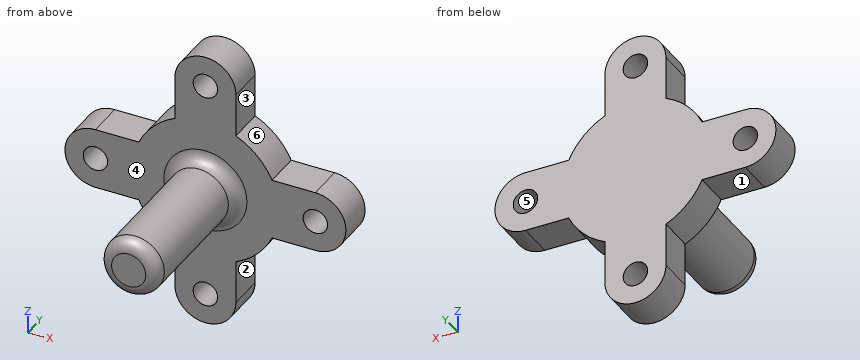
```python
from build123d import *

# Parameters (mm, degrees)
SKETCH1_R           = 5
BOSS_EXTRUDE1_DEPTH = 7.5
SKETCH2_R           = 12
BOSS_EXTRUDE2_DEPTH = 60
FILLET1_R           = 5
SCALE1_SCALE        = 0.6


with BuildPart() as part:
    # Sketch1 → Boss-Extrude1 (new body, symmetric)
    with BuildSketch(Plane(origin=(0, 0, 0), x_dir=(1, 0, 0), z_dir=(0, 1, 0))):
        with BuildLine():
            Line((12.5, 45.011324124), (12.5, 27.271780287))
            ThreePointArc((12.5, 27.271780287), (21.213203436, 21.213203436), (27.271780287, 12.5))
            Line((27.271780287, 12.5), (45, 12.5))
            ThreePointArc((45, 12.5), (57.511322842, 0.00566206), (45.011324124, -12.5))
            Line((45.011324124, -12.5), (27.271780287, -12.5))
            ThreePointArc((27.271780287, -12.5), (21.213203436, -21.213203436), (12.5, -27.271780287))
            Line((12.5, -27.271780287), (12.5, -45))
            ThreePointArc((12.5, -45), (0.00566206, -57.511322842), (-12.5, -45.011324124))
            Line((-12.5, -45.011324124), (-12.5, -27.271780287))
            ThreePointArc((-12.5, -27.271780287), (-21.213203436, -21.213203436), (-27.271780287, -12.5))
            Line((-27.271780287, -12.5), (-45, -12.5))
            ThreePointArc((-45, -12.5), (-57.511322842, -0.00566206), (-45.011324124, 12.5))
            Line((-45.011324124, 12.5), (-27.271780287, 12.5))
            ThreePointArc((-27.271780287, 12.5), (-21.213203436, 21.213203436), (-12.5, 27.271780287))
            Line((-12.5, 27.271780287), (-12.5, 45))
            ThreePointArc((-12.5, 45), (-0.00566206, 57.511322842), (12.5, 45.011324124))
        make_face()
        with Locations((0, 45.011324124)):
            Circle(SKETCH1_R, mode=Mode.SUBTRACT)
        with Locations((45.011324124, 0)):
            Circle(SKETCH1_R, mode=Mode.SUBTRACT)
        with Locations((0, -45.011324124)):
            Circle(SKETCH1_R, mode=Mode.SUBTRACT)
        with Locations((-45.011324124, 0)):
            Circle(SKETCH1_R, mode=Mode.SUBTRACT)
    extrude(amount=BOSS_EXTRUDE1_DEPTH, both=True)

    # Sketch2 → Boss-Extrude2 (add)
    with BuildSketch(Plane.XZ.offset(7.5)):
        Circle(SKETCH2_R)
    extrude(amount=BOSS_EXTRUDE2_DEPTH)

    # Fillet1
    fillet1_edges = [part.edges().sort_by_distance(p)[0] for p in [
        (-12, -7.5, 0),
        (-12, -67.5, 0),
    ]]
    fillet(fillet1_edges, radius=FILLET1_R)


with BuildPart() as part_1:
    # Scale1: scaled about (0, -9.636129327, 0)
    add(part.part.scale(SCALE1_SCALE).moved(Location((0, -3.854451731, 0))))


solid = part_1.part
```
Check sheet for the modelled part. Datum: model origin and axes. Units: mm. Face numbers are marked on the shaded views. A direction names the side the tool comes from. Round coordinates to 2 decimals unless told otherwise and drop trailing zeros. Loops run counter-clockwise (first coordinate to the right, second up) from the corner with the lowest first, then second, coordinate; pieces in that order, holes last. Notation, with made-up numbers: M 36,19.25 L 40,19.25 A20 cw 40,49.25 Z; hole C -2.5,79.25 d11. An arc over 180 degrees is marked long. Answer as a JSON object with one key per item and string values.
1. Section check B-B (z = -25.5). Record the boundary of the cut face in (x, y).
Reply:
{"outline": "M -7.5,-8.35 L -2.59,-8.35 L -2.59,0.65 L -7.5,0.65 Z; M 2.59,-8.35 L 7.5,-8.35 L 7.5,0.65 L 2.59,0.65 Z"}
2. Scan lines: line 1 (Z direction, x = 0, y = -4.75); line 2 (X direction, y = -1, z = 2). Record each from-to range of solid material in increasing order.
Reply:
{"line 1": "z = -34.51 to -30.01, -24.01 to 24.01, 30.01 to 34.51", "line 2": "x = -34.24 to -29.24, -24.77 to 24.77, 29.24 to 34.24"}
3. Access from +Z, -Z, +X, -X, +Y, -Y to the whole of each face (thin tool, end or side, straight path). Record for the marked faces 1, 2 and 3.
Reply:
{"face 1": "-Z, -X, +Y, -Y", "face 2": "-Z, +X, +Y, -Y", "face 3": "+Z, +X, +Y, -Y"}
4. Section check D-D (y = -15). Record the boundary of the cut face in (x, z).
Reply:
{"outline": "C 0,0 d14.4"}
5. Mould release check, pull along X, two halves, no side actions. Record for the marked faces 4, 5 and 6: pulls with the +X half, pulls with the -X half, needs draft (parallel to the pull), parting line crosses it, or undercut.
Reply:
{"face 4": "needs draft", "face 5": "undercut", "face 6": "pulls with the +X half"}
6. Section check A-A (x = 0). Record the boundary of the cut face in (y, z).
Reply:
{"outline": "M -44.35,-4.2 A3 ccw -41.35,-7.2 L -11.35,-7.2 A3 cw -8.35,-10.2 L -8.35,-24.01 L 0.65,-24.01 L 0.65,24.01 L -8.35,24.01 L -8.35,10.2 A3 cw -11.35,7.2 L -41.35,7.2 A3 ccw -44.35,4.2 Z; M -8.35,-34.51 L 0.65,-34.51 L 0.65,-30.01 L -8.35,-30.01 Z; M -8.35,30.01 L 0.65,30.01 L 0.65,34.51 L -8.35,34.51 Z"}
7. Section check C-C (z = 0). Record the boundary of the cut face in (x, y), plus the area to 3 significant figures.
Reply:
{"outline": "M -34.51,-8.35 L -30.01,-8.35 L -30.01,0.65 L -34.51,0.65 Z; M -24.01,-8.35 L -10.2,-8.35 A3 cw -7.2,-11.35 L -7.2,-41.35 A3 ccw -4.2,-44.35 L 4.2,-44.35 A3 ccw 7.2,-41.35 L 7.2,-11.35 A3 cw 10.2,-8.35 L 24.01,-8.35 L 24.01,0.65 L -24.01,0.65 Z; M 30.01,-8.35 L 34.51,-8.35 L 34.51,0.65 L 30.01,0.65 Z", "area": "1,030 mm²"}
8. Gauge pin test, flat ends, axial feed: P1, Ø4.5, axis at x = -22, y = -3, coming from the -Z side; P2, Ø6, axis at y = -12, z = 3.5, coming from the +X side; P3, Ø3, axis at x = 3, y = -27.5, coming from the -Z side; P4, Ø7, axis at x = 0, z = 27.01, coming from the +Y side. Record the tip position at first contact, or that the pin passes through.
Reply:
{"P1": "stops at z = -7.5", "P2": "stops at x = 7.75", "P3": "stops at z = -7.04", "P4": "stops at y = 0.65"}
